Can you work these out from the model? Positions are in its coordinate system, mm. Face numbers are marked on the shaded views. A direction names the side the tool comes from. Give positions to 0.01 mm unless a question says otherwise; leave off trailing zeros. Loops run counter-clockwise (first coordinate to the right, second up) from the corner with the lowest first, then second, coordinate; pieces in that order, holes last.
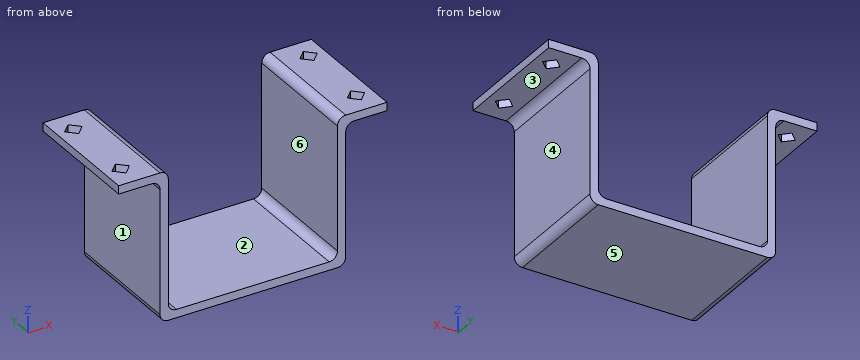
from build123d import *

# Parameters (mm, degrees)
SKETCH1_W           = 57.15
SKETCH1_H           = 38.1
BOSS_EXTRUDE1_DEPTH = 2.54
SKETCH2_W           = 2.54
SKETCH2_H           = 38.1
BOSS_EXTRUDE2_DEPTH = 43.18
SKETCH3_W           = 2.54
SKETCH3_H           = 38.1
BOSS_EXTRUDE3_DEPTH = 12.7
SKETCH4_W           = 2.54
SKETCH4_H           = 38.1
BOSS_EXTRUDE4_DEPTH = 12.7
FILLET1_R           = 2.54
CUT_EXTRUDE1_DEPTH  = 91.527039607


with BuildPart() as part:
    # Sketch1 → Boss-Extrude1 (new body)
    with BuildSketch(Plane.XY):
        with Locations((28.575, 19.05)):
            Rectangle(SKETCH1_W, SKETCH1_H)
    extrude(amount=BOSS_EXTRUDE1_DEPTH)

    # Sketch2 → Boss-Extrude2 (add)
    with BuildSketch(Plane.XY.offset(2.54)):
        with Locations((1.27, 19.05)):
            Rectangle(SKETCH2_W, SKETCH2_H)
        with Locations((55.88, 19.05)):
            Rectangle(SKETCH2_W, SKETCH2_H)
    extrude(amount=BOSS_EXTRUDE2_DEPTH)

    # Sketch3 → Boss-Extrude3 (add)
    with BuildSketch(Plane(origin=(57.15, 0, 0), x_dir=(0, 0, -1), z_dir=(1, 0, 0))):
        with Locations((-44.45, 19.05)):
            Rectangle(SKETCH3_W, SKETCH3_H)
    extrude(amount=BOSS_EXTRUDE3_DEPTH)

    # Sketch4 → Boss-Extrude4 (add)
    with BuildSketch(Plane.ZY):
        with Locations((44.45, 19.05)):
            Rectangle(SKETCH4_W, SKETCH4_H)
    extrude(amount=BOSS_EXTRUDE4_DEPTH)

    # Fillet1
    fillet1_edges = [part.edges().sort_by_distance(p)[0] for p in [
        (2.54, 19.05, 2.54),
        (2.54, 19.05, 45.72),
        (54.61, 19.05, 2.54),
        (54.61, 19.05, 45.72),
        (57.15, 19.05, 43.18),
        (57.15, 19.05, 0),
        (0, 19.05, 43.18),
        (0, 19.05, 0),
    ]]
    fillet(fillet1_edges, radius=FILLET1_R)

    # Sketch5 → Cut-Extrude1 (cut, through all)
    with BuildSketch(Plane(origin=(0, 0, 43.18), x_dir=(-1, 0, 0), z_dir=(0, 0, -1))):
        Polygon((-64.77, 33.800232648), (-67.446116324, 31.124116324), (-64.77, 28.448), (-62.093883676, 31.124116324), align=None)
        Polygon((-64.77, 9.987732648), (-67.446116324, 7.311616324), (-64.77, 4.6355), (-62.093883676, 7.311616324), align=None)
        Polygon((4.943883676, 7.311616324), (7.62, 9.987732648), (10.296116324, 7.311616324), (7.62, 4.6355), align=None)
        Polygon((4.943883676, 31.124116324), (7.62, 33.800232648), (10.296116324, 31.124116324), (7.62, 28.448), align=None)
    extrude(amount=-CUT_EXTRUDE1_DEPTH, mode=Mode.SUBTRACT)


solid = part.part
(1) Which directions (+Z, -Z, +X, -X, +Y, -Y) give clear straight access to the entire face, cutting with the end or side of a thin tool? Please do the marked faces 1, 2 and 3.
Returned:
face 1: -Z, -X, +Y, -Y
face 2: +Z, +Y, -Y
face 3: -Z, +X, +Y, -Y
(2) Will these pins go through, and if not, where does the flat tip stop? P1, Ø1.5, axis at y = 27.5, z = 12, coming from the -X side; P2, Ø5, axis at x = -9, y = 16.5, coming from the -Z side; P3, Ø8, axis at x = -3.5, y = 10, coming from the -Z side.
Returned:
P1: stops at x = 0
P2: stops at z = 43.18
P3: stops at z = 1.03
(3) Suppose I cut it at C-C on x = 63. List the corners of the cut face in (y, z) for me, plus the area to 3 significant figures.
Returned:
outline: (0, 43.18) - (6.41, 43.18) - (6.41, 45.72) - (0, 45.72) - close; (8.22, 43.18) - (30.22, 43.18) - (30.22, 45.72) - (8.22, 45.72) - close; (32.03, 43.18) - (38.1, 43.18) - (38.1, 45.72) - (32.03, 45.72) - close
area: 87.6 mm2
(4) Thinking about a two-plate mould opening in X: for the marked faces 4, 5 and 6, which applies, pulls with the +X half, pulls with the -X half, needs draft (parallel to the pull), parting line crosses it, or undercut?
Returned:
face 4: pulls with the +X half
face 5: needs draft
face 6: undercut
(5) Suppose I cut it at D-D on y = 32. List the corners of the cut face in (x, z) for me, plus the area to 3 significant figures.
Returned:
outline: (-12.7, 43.18) - (-9.42, 43.18) - (-9.42, 45.72) - (-12.7, 45.72) - close; (-5.82, 43.18) - (-2.54, 43.18) arc R2.54 cw to (0, 40.64) - (0, 2.54) arc R2.54 ccw to (2.54, 0) - (54.61, 0) arc R2.54 ccw to (57.15, 2.54) - (57.15, 40.64) arc R2.54 cw to (59.69, 43.18) - (62.97, 43.18) - (62.97, 45.72) - (57.15, 45.72) arc R2.54 ccw to (54.61, 43.18) - (54.61, 5.08) arc R2.54 cw to (52.07, 2.54) - (5.08, 2.54) arc R2.54 cw to (2.54, 5.08) - (2.54, 43.18) arc R2.54 ccw to (0, 45.72) - (-5.82, 45.72) - close; (66.57, 43.18) - (69.85, 43.18) - (69.85, 45.72) - (66.57, 45.72) - close
area: 411 mm2
(6) Please list where these lines run through material, in increasing order: probe 1 along X at (y, z) = (14, 13); probe 2 along Z at (x, y) = (22, 28.5); probe 3 along Z at (x, y) = (-3.5, 19.5).
Returned:
probe 1: x = 0 to 2.54, 54.61 to 57.15
probe 2: z = 0 to 2.54
probe 3: z = 43.18 to 45.72
(7) Suppose I cut it at A-A on z = 19. List the corners of the cut face in (x, y) for me.
Returned:
outline: (0, 0) - (2.54, 0) - (2.54, 38.1) - (0, 38.1) - close; (54.61, 0) - (57.15, 0) - (57.15, 38.1) - (54.61, 38.1) - close
(8) Suppose I cut it at B-B on y = 17. List the corners of the cut face in (x, z) for me, plus the area to 3 significant figures.
Returned:
outline: (-12.7, 43.18) - (-2.54, 43.18) arc R2.54 cw to (0, 40.64) - (0, 2.54) arc R2.54 ccw to (2.54, 0) - (54.61, 0) arc R2.54 ccw to (57.15, 2.54) - (57.15, 40.64) arc R2.54 cw to (59.69, 43.18) - (69.85, 43.18) - (69.85, 45.72) - (57.15, 45.72) arc R2.54 ccw to (54.61, 43.18) - (54.61, 5.08) arc R2.54 cw to (52.07, 2.54) - (5.08, 2.54) arc R2.54 cw to (2.54, 5.08) - (2.54, 43.18) arc R2.54 ccw to (0, 45.72) - (-12.7, 45.72) - close
area: 429 mm2
